from build123d import *

# Parameters (mm, degrees)
F0_R     = 5.75
F1_DEPTH = 2.5
F2_DEPTH = 18.5
F3_DEPTH = 6.5
F4_DEPTH = 1.5


with BuildPart() as f1:
    # F0 (on Top) → F1 (new body)
    with BuildSketch(Plane.XY):
        Circle(F0_R)
        with BuildLine():
            ThreePointArc((5.2037929302, 0.6950101723), (5.2384354956, 0.3482722473), (5.25, 0))
            ThreePointArc((5.25, 0), (4.3624820917, -2.9208303614), (2, -4.8541219597))
            ThreePointArc((2, -4.8541219597), (1.6540858778, -4.9826197837), (1.3, -5.0865017448))
            ThreePointArc((1.3, -5.0865017448), (0, -5.25), (-1.3, -5.0865017448))
            ThreePointArc((-1.3, -5.0865017448), (-1.6540858778, -4.9826197837), (-2, -4.8541219597))
            ThreePointArc((-2, -4.8541219597), (-4.5466333699, -2.625), (-5.2037929302, 0.6950101723))
            ThreePointArc((-5.2037929302, 0.6950101723), (-5.142118249, 1.0588295016), (-5.0550397274, 1.4174178475))
            ThreePointArc((-5.0550397274, 1.4174178475), (-4.5466333699, 2.625), (-3.7550397274, 3.6690838973))
            ThreePointArc((-3.7550397274, 3.6690838973), (-3.4880323712, 3.9237902821), (-3.2037929302, 4.1591117874))
            ThreePointArc((-3.2037929302, 4.1591117874), (0, 5.25), (3.2037929302, 4.1591117874))
            ThreePointArc((3.2037929302, 4.1591117874), (3.4880323712, 3.9237902821), (3.7550397274, 3.6690838973))
            ThreePointArc((3.7550397274, 3.6690838973), (4.5466333699, 2.625), (5.0550397274, 1.4174178475))
            ThreePointArc((5.0550397274, 1.4174178475), (5.142118249, 1.0588295016), (5.2037929302, 0.6950101723))
        make_face(mode=Mode.SUBTRACT)
        with BuildLine():
            Line((2, -1.1547005384), (5.2037929302, 0.6950101723))
            ThreePointArc((5.2037929302, 0.6950101723), (5.142118249, 1.0588295016), (5.0550397274, 1.4174178475))
            Line((5.0550397274, 1.4174178475), (2.8899762179, 0.1674178475))
            ThreePointArc((2.8899762179, 0.1674178475), (1.7668965617, 1.0201182055), (1.5899762179, 2.4190838973))
            Line((1.5899762179, 2.4190838973), (3.7550397274, 3.6690838973))
            ThreePointArc((3.7550397274, 3.6690838973), (3.4880323712, 3.9237902821), (3.2037929302, 4.1591117874))
            Line((3.2037929302, 4.1591117874), (0, 2.3094010768))
            Line((0, 2.3094010768), (-3.2037929302, 4.1591117874))
            ThreePointArc((-3.2037929302, 4.1591117874), (-3.4880323712, 3.9237902821), (-3.7550397274, 3.6690838973))
            Line((-3.7550397274, 3.6690838973), (-1.5899762179, 2.4190838973))
            ThreePointArc((-1.5899762179, 2.4190838973), (-1.7668965617, 1.0201182055), (-2.8899762179, 0.1674178475))
            Line((-2.8899762179, 0.1674178475), (-5.0550397274, 1.4174178475))
            ThreePointArc((-5.0550397274, 1.4174178475), (-5.142118249, 1.0588295016), (-5.2037929302, 0.6950101723))
            Line((-5.2037929302, 0.6950101723), (-2, -1.1547005384))
            Line((-2, -1.1547005384), (-2, -4.8541219597))
            ThreePointArc((-2, -4.8541219597), (-1.6540858778, -4.9826197837), (-1.3, -5.0865017448))
            Line((-1.3, -5.0865017448), (-1.3, -2.5865017448))
            ThreePointArc((-1.3, -2.5865017448), (0, -2.0402364111), (1.3, -2.5865017448))
            Line((1.3, -2.5865017448), (1.3, -5.0865017448))
            ThreePointArc((1.3, -5.0865017448), (1.6540858778, -4.9826197837), (2, -4.8541219597))
            Line((2, -4.8541219597), (2, -1.1547005384))
        make_face()
        Polygon((-1.3, -0.7505553499), (0, 1.5011106999), (1.3, -0.7505553499), align=None, mode=Mode.SUBTRACT)
    extrude(amount=F1_DEPTH)

    # F0 (on Top) → F2 (join)
    with BuildSketch(Plane.XY):
        Polygon((1.3, -0.7505553499), (0, 1.5011106999), (-1.3, -0.7505553499), align=None)
        Polygon((-0.8, -0.4618802154), (0, 0.9237604307), (0.8, -0.4618802154), align=None, mode=Mode.SUBTRACT)
    extrude(amount=F2_DEPTH)

    # F0 (on Top) → F3 (join)
    with BuildSketch(Plane.XY):
        Circle(F0_R)
        with BuildLine():
            ThreePointArc((5.2037929302, 0.6950101723), (5.2384354956, 0.3482722473), (5.25, 0))
            ThreePointArc((5.25, 0), (4.3624820917, -2.9208303614), (2, -4.8541219597))
            ThreePointArc((2, -4.8541219597), (1.6540858778, -4.9826197837), (1.3, -5.0865017448))
            ThreePointArc((1.3, -5.0865017448), (0, -5.25), (-1.3, -5.0865017448))
            ThreePointArc((-1.3, -5.0865017448), (-1.6540858778, -4.9826197837), (-2, -4.8541219597))
            ThreePointArc((-2, -4.8541219597), (-4.5466333699, -2.625), (-5.2037929302, 0.6950101723))
            ThreePointArc((-5.2037929302, 0.6950101723), (-5.142118249, 1.0588295016), (-5.0550397274, 1.4174178475))
            ThreePointArc((-5.0550397274, 1.4174178475), (-4.5466333699, 2.625), (-3.7550397274, 3.6690838973))
            ThreePointArc((-3.7550397274, 3.6690838973), (-3.4880323712, 3.9237902821), (-3.2037929302, 4.1591117874))
            ThreePointArc((-3.2037929302, 4.1591117874), (0, 5.25), (3.2037929302, 4.1591117874))
            ThreePointArc((3.2037929302, 4.1591117874), (3.4880323712, 3.9237902821), (3.7550397274, 3.6690838973))
            ThreePointArc((3.7550397274, 3.6690838973), (4.5466333699, 2.625), (5.0550397274, 1.4174178475))
            ThreePointArc((5.0550397274, 1.4174178475), (5.142118249, 1.0588295016), (5.2037929302, 0.6950101723))
        make_face(mode=Mode.SUBTRACT)
    extrude(amount=-F3_DEPTH)

    # F0 (on Top) → F4 (join)
    with BuildSketch(Plane.XY):
        with BuildLine():
            Line((2, -1.1547005384), (5.2037929302, 0.6950101723))
            ThreePointArc((5.2037929302, 0.6950101723), (5.142118249, 1.0588295016), (5.0550397274, 1.4174178475))
            Line((5.0550397274, 1.4174178475), (2.8899762179, 0.1674178475))
            ThreePointArc((2.8899762179, 0.1674178475), (1.7668965617, 1.0201182055), (1.5899762179, 2.4190838973))
            Line((1.5899762179, 2.4190838973), (3.7550397274, 3.6690838973))
            ThreePointArc((3.7550397274, 3.6690838973), (3.4880323712, 3.9237902821), (3.2037929302, 4.1591117874))
            Line((3.2037929302, 4.1591117874), (0, 2.3094010768))
            Line((0, 2.3094010768), (-3.2037929302, 4.1591117874))
            ThreePointArc((-3.2037929302, 4.1591117874), (-3.4880323712, 3.9237902821), (-3.7550397274, 3.6690838973))
            Line((-3.7550397274, 3.6690838973), (-1.5899762179, 2.4190838973))
            ThreePointArc((-1.5899762179, 2.4190838973), (-1.7668965617, 1.0201182055), (-2.8899762179, 0.1674178475))
            Line((-2.8899762179, 0.1674178475), (-5.0550397274, 1.4174178475))
            ThreePointArc((-5.0550397274, 1.4174178475), (-5.142118249, 1.0588295016), (-5.2037929302, 0.6950101723))
            Line((-5.2037929302, 0.6950101723), (-2, -1.1547005384))
            Line((-2, -1.1547005384), (-2, -4.8541219597))
            ThreePointArc((-2, -4.8541219597), (-1.6540858778, -4.9826197837), (-1.3, -5.0865017448))
            Line((-1.3, -5.0865017448), (-1.3, -2.5865017448))
            ThreePointArc((-1.3, -2.5865017448), (0, -2.0402364111), (1.3, -2.5865017448))
            Line((1.3, -2.5865017448), (1.3, -5.0865017448))
            ThreePointArc((1.3, -5.0865017448), (1.6540858778, -4.9826197837), (2, -4.8541219597))
            Line((2, -4.8541219597), (2, -1.1547005384))
        make_face()
        Polygon((-1.3, -0.7505553499), (0, 1.5011106999), (1.3, -0.7505553499), align=None, mode=Mode.SUBTRACT)
    extrude(amount=-F4_DEPTH)


solid = f1.part
Design review of the part built by this model. Coordinates are the model's own, in mm. A direction names the side the tool comes from. Coordinates: 2 decimals unless noted, no trailing zeros. Write each loop counter-clockwise with the first axis right and the second up, starting at its lowest first coordinate (ties: lowest second). Pieces come first, ordered by that corner, then holes. Notation, with made-up numbers: (-29, 61) - (20, 61) arc R22 cw to (20, 81) - close; hole circle Ø2 at (22, -33). An arc over 180 degrees is marked (long way). Use one line per item in the form item = value.
Q1. Consider section D-D (z = 9.25). Write out the cut boundary in (x, y), plus the area to 3 significant figures.
Taken from the geometry:
outline = (-1.3, -0.75) - (1.3, -0.75) - (0, 1.5) - close; hole (-0.8, -0.46) - (0.8, -0.46) - (0, 0.92) - close
area = 1.82 mm^2
Q2. Consider section A-A (z = 1.5). Write out the cut boundary in (x, y), plus the area to 3 significant figures.
Taken from the geometry:
outline = circle Ø11.5 at (0, 0); hole (-5.2, 0.7) arc R5.25 ccw to (-2, -4.85) - (-2, -1.15) - close; hole (-5.06, 1.42) - (-2.89, 0.17) arc R1.82 ccw to (-1.59, 2.42) - (-3.76, 3.67) arc R5.25 ccw to start; hole (-3.2, 4.16) - (0, 2.31) - (3.2, 4.16) arc R5.25 ccw to start; hole (-1.3, -5.09) arc R5.25 ccw to (1.3, -5.09) - (1.3, -2.59) arc R1.82 ccw to (-1.3, -2.59) - close; hole (-0.8, -0.46) - (0.8, -0.46) - (0, 0.92) - close; hole (1.59, 2.42) arc R1.82 ccw to (2.89, 0.17) - (5.06, 1.42) arc R5.25 ccw to (3.76, 3.67) - close; hole (2, -4.85) arc R5.25 ccw to (5.2, 0.7) - (2, -1.15) - close
area = 47.4 mm^2
Q3. Insertion check: pin 1 Ø1.1 at (y, z) = (-4, 0) entering from +X; pin 2 Ø4.5 at (x, y) = (0, 1) entering from -Z; pin 3 Ø5 at (y, z) = (3, 13) entering from -X. Each pin has a flat end and moves straight along its axis. Give the tip position at first contact, or say it passes through.
Taken from the geometry:
pin_1 = 4.6
pin_2 = -1.5
pin_3 = -0.58
Q4. Consider section C-C (y = -3.75). Write out the cut boundary in (x, z).
Taken from the geometry:
outline = (-4.36, -6.5) - (-3.67, -6.5) - (-3.67, 2.5) - (-4.36, 2.5) - close; (-2, -1.5) - (-1.3, -1.5) - (-1.3, 2.5) - (-2, 2.5) - close; (1.3, -1.5) - (2, -1.5) - (2, 2.5) - (1.3, 2.5) - close; (3.67, -6.5) - (4.36, -6.5) - (4.36, 2.5) - (3.67, 2.5) - close
Q5. Consider section B-B (x = 4.25). Write out the cut boundary in (y, z).
Taken from the geometry:
outline = (-3.87, -6.5) - (-3.08, -6.5) - (-3.08, 2.5) - (-3.87, 2.5) - close; (0.14, -1.5) - (0.95, -1.5) - (0.95, 2.5) - (0.14, 2.5) - close; (3.08, -6.5) - (3.87, -6.5) - (3.87, 2.5) - (3.08, 2.5) - close
Q6. The part is to be moulded in two halves that separate along Y. For faces 3 (the flat face through (0, -0.751, 10)), 4 (the flat face through (-2, -3, 1)), 5 (the cylindrical face through (-0.75, 5.7, -1.94)), 6 (the flat face through (-0.66, 0.36, -0.74)), say which applies: +Y half, -Y half, draft (parallel to the pull), parting line (faces both ways), or undercut.
Taken from the geometry:
face_3 = -Y half
face_4 = undercut
face_5 = parting line
face_6 = undercut
Q7. For probe 1 along Z at (x, y) = (1.5, -2.25); probe 2 along Y at (x, z) = (-0.5, 3.5); probe 3 along Y at (x, z) = (1.25, -4.5), list the stretches that pass through material, from the lowest coordinate up.
Taken from the geometry:
probe_1 = -1.5 to 2.5
probe_2 = -0.75 to -0.46, 0.06 to 0.64
probe_3 = -5.61 to -5.1, 5.1 to 5.61
Q8. Machinability: for faces 1 (the flat face through (-3.957, 0.784, 0.528)), 2 (the flat face through (0, -0.751, -1)), which of the approach directions +Z, -Z, +X, -X, +Y, -Y give a long, thin tool a straight path to every point of the face, cutting with its end or side? Answer none if there is none.
Taken from the geometry:
face_1 = +Z, -Z
face_2 = -Z
